```python
from build123d import *

# Parameters (mm, degrees)
BOSS_EXTRUDE1_DEPTH            = 50
SKETCH2_R                      = 7.6
SKETCH2_R_2                    = 4.75
SKETCH2_R_3                    = 1.55
SKETCH2_R_4                    = 1.05
CUT_EXTRUDE1_DEPTH             = 116.876011322
CUT_EXTRUDE2_DEPTH             = 5.5
SKETCH4_R                      = 11
CUT_EXTRUDE3_DEPTH             = 29
CUT_EXTRUDE4_DEPTH             = 5
CUT_EXTRUDE5_DEPTH             = 2.5
SKETCH7_R                      = 4.1
SKETCH7_R_2                    = 1.6
SKETCH7_W                      = 12
SKETCH7_H                      = 24
CUT_EXTRUDE6_DEPTH             = 116.876011322
CUT_EXTRUDE7_DEPTH             = 35
SKETCH9_W                      = 17
SKETCH9_H                      = 16
CUT_EXTRUDE8_DEPTH             = 48
CUT_EXTRUDE9_REACH             = 117.876
SKETCH10_W                     = 37
SKETCH10_H                     = 8
CUT_EXTRUDE9_DIRECTION_2_DEPTH = 116.876011322
CUT_EXTRUDE10_REACH            = 115.716
SKETCH11_W                     = 18.5
SKETCH11_H                     = 8
FILLET1_R                      = 8


with BuildPart() as part:
    # Sketch1 → Boss-Extrude1 (new body)
    with BuildSketch(Plane(origin=(0, 0, 0), x_dir=(0, 0, -1), z_dir=(1, 0, 0))):
        Polygon((0, 0), (0, 30), (5, 30), (5, 35), (-98.5, 35), (-98.5, 0), align=None)
    extrude(amount=BOSS_EXTRUDE1_DEPTH)

    # Sketch2 → Cut-Extrude1 (cut, through all)
    with BuildSketch(Plane(origin=(0, 35, 0), x_dir=(1, 0, 0), z_dir=(0, 1, 0))):
        with Locations(Location((36.5, -48.5, 0), (0, 0, 270))):
            Circle(SKETCH2_R)
        with Locations(Location((13.5, -48.5, 0), (0, 0, 270))):
            Circle(SKETCH2_R_2)
        with Locations(Location((36.5, -36.25, 0), (0, 0, 270))):
            Circle(SKETCH2_R_3)
        with Locations(Location((36.5, -60.75, 0), (0, 0, 270))):
            Circle(SKETCH2_R_3)
        with Locations(Location((19.156854249, -42.843145751, 0), (0, 0, 270))):
            Circle(SKETCH2_R_4)
        with Locations(Location((19.156854249, -54.156854249, 0), (0, 0, 270))):
            Circle(SKETCH2_R_4)
        with Locations(Location((7.843145751, -54.156854249, 0), (0, 0, 270))):
            Circle(SKETCH2_R_4)
        with Locations(Location((7.843145751, -42.843145751, 0), (0, 0, 270))):
            Circle(SKETCH2_R_4)
    extrude(amount=-CUT_EXTRUDE1_DEPTH, mode=Mode.SUBTRACT)

    # Sketch3 → Cut-Extrude2 (cut)
    with BuildSketch(Plane(origin=(0, 35, 0), x_dir=(1, 0, 0), z_dir=(0, 1, 0))):
        with BuildLine():
            Line((25.9, -36.381831822), (25.9, -60.618168178))
            ThreePointArc((25.9, -60.618168178), (36.5, -64.6), (47.1, -60.618168178))
            Line((47.1, -60.618168178), (47.1, -36.381831822))
            ThreePointArc((47.1, -36.381831822), (36.5, -32.4), (25.9, -36.381831822))
        make_face()
    extrude(amount=-CUT_EXTRUDE2_DEPTH, mode=Mode.SUBTRACT)

    # Sketch4 → Cut-Extrude3 (cut)
    with BuildSketch(Plane.XZ):
        with Locations(Location((13.5, 48.5, 0), (0, 0, 270))):
            Circle(SKETCH4_R)
    extrude(amount=-CUT_EXTRUDE3_DEPTH, mode=Mode.SUBTRACT)

    # Sketch5 → Cut-Extrude4 (cut)
    with BuildSketch(Plane.XZ):
        Polygon((39.725, 60.75), (38.1125, 63.542931927), (34.8875, 63.542931927), (33.275, 60.75), (34.8875, 57.957068073), (38.1125, 57.957068073), align=None)
        Polygon((38.1125, 39.042931927), (34.8875, 39.042931927), (33.275, 36.25), (34.8875, 33.457068073), (38.1125, 33.457068073), (39.725, 36.25), align=None)
    extrude(amount=-CUT_EXTRUDE4_DEPTH, mode=Mode.SUBTRACT)

    # Sketch6 → Cut-Extrude5 (cut)
    with BuildSketch(Plane(origin=(0, 35, 0), x_dir=(1, 0, 0), z_dir=(0, 1, 0))):
        Polygon((21.388142908, -42.245273756), (19.754726244, -40.611857092), (17.523437585, -41.209729086), (16.925565591, -43.441017745), (18.558982255, -45.074434409), (20.790270914, -44.476562415), align=None)
        Polygon((21.388142908, -54.754726244), (20.790270914, -52.523437585), (18.558982255, -51.925565591), (16.925565591, -53.558982255), (17.523437585, -55.790270914), (19.754726244, -56.388142908), align=None)
        Polygon((7.245273756, -56.388142908), (9.476562415, -55.790270914), (10.074434409, -53.558982255), (8.441017745, -51.925565591), (6.209729086, -52.523437585), (5.611857092, -54.754726244), align=None)
        Polygon((5.611857092, -42.245273756), (6.209729086, -44.476562415), (8.441017745, -45.074434409), (10.074434409, -43.441017745), (9.476562415, -41.209729086), (7.245273756, -40.611857092), align=None)
    extrude(amount=-CUT_EXTRUDE5_DEPTH, mode=Mode.SUBTRACT)

    # Sketch7 → Cut-Extrude6 (cut, through all)
    with BuildSketch(Plane(origin=(50, 0, 0), x_dir=(0, 0, -1), z_dir=(1, 0, 0))):
        with Locations((-8.5, 26)):
            Circle(SKETCH7_R)
        with Locations((-88.5, 26)):
            Circle(SKETCH7_R)
        with Locations((-88.5, 16)):
            Circle(SKETCH7_R_2)
        with Locations((-8.5, 16)):
            Circle(SKETCH7_R_2)
        with Locations((-68.5, 30)):
            Circle(SKETCH7_R_2)
        with Locations((-68.5, 5)):
            Circle(SKETCH7_R_2)
        with Locations((-24, 15)):
            Rectangle(SKETCH7_W, SKETCH7_H)
    extrude(amount=-CUT_EXTRUDE6_DEPTH, mode=Mode.SUBTRACT)

    # Sketch8 → Cut-Extrude7 (cut)
    with BuildSketch(Plane.ZY):
        Polygon((11.725, 16), (10.1125, 18.792931927), (6.8875, 18.792931927), (5.275, 16), (6.8875, 13.207068073), (10.1125, 13.207068073), align=None)
        Polygon((65.275, 30), (66.8875, 27.207068073), (70.1125, 27.207068073), (71.725, 30), (70.1125, 32.792931927), (66.8875, 32.792931927), align=None)
        Polygon((65.275, 5), (66.8875, 2.207068073), (70.1125, 2.207068073), (71.725, 5), (70.1125, 7.792931927), (66.8875, 7.792931927), align=None)
        Polygon((85.275, 16), (86.8875, 13.207068073), (90.1125, 13.207068073), (91.725, 16), (90.1125, 18.792931927), (86.8875, 18.792931927), align=None)
    extrude(amount=-CUT_EXTRUDE7_DEPTH, mode=Mode.SUBTRACT)

    # Sketch9 → Cut-Extrude8 (cut)
    with BuildSketch(Plane(origin=(50, 0, 0), x_dir=(0, 0, -1), z_dir=(1, 0, 0))):
        with Locations((-24, 13)):
            Rectangle(SKETCH9_W, SKETCH9_H)
    extrude(amount=-CUT_EXTRUDE8_DEPTH, mode=Mode.SUBTRACT)

    # Sketch10 → Cut-Extrude9 (cut, up to next)
    with BuildSketch(Plane.XZ, mode=Mode.PRIVATE) as cut_extrude9_sk1:
        with Locations((25, 24)):
            Rectangle(SKETCH10_W, SKETCH10_H)
    cut_extrude9_tool1 = extrude(cut_extrude9_sk1.sketch, amount=-CUT_EXTRUDE9_REACH, mode=Mode.PRIVATE) & part.part
    add(cut_extrude9_tool1.solids().sort_by_distance((25, 0, 24))[0], mode=Mode.SUBTRACT)

    # Sketch10 → Cut-Extrude9 direction 2 (cut)
    with BuildSketch(Plane.XZ):
        with Locations((25, 24)):
            Rectangle(SKETCH10_W, SKETCH10_H)
    extrude(amount=CUT_EXTRUDE9_DIRECTION_2_DEPTH, mode=Mode.SUBTRACT)

    # Sketch11 → Cut-Extrude10 (cut, up to next)
    with BuildSketch(Plane.XZ.offset(-27), mode=Mode.PRIVATE) as cut_extrude10_sk1:
        with Locations((15.75, 24)):
            Rectangle(SKETCH11_W, SKETCH11_H)
    cut_extrude10_tool1 = extrude(cut_extrude10_sk1.sketch, amount=-CUT_EXTRUDE10_REACH, mode=Mode.PRIVATE) & part.part
    add(cut_extrude10_tool1.solids().sort_by_distance((15.75, 27, 24))[0], mode=Mode.SUBTRACT)

    # Fillet1
    fillet1_edges = [part.edges().sort_by_distance(p)[0] for p in [
        (25, 35, 98.5),
    ]]
    fillet(fillet1_edges, radius=FILLET1_R)


solid = part.part
```
Design review of the part built by this model. Coordinates are the model's own, in mm. A direction names the side the tool comes from. Round coordinates to 2 decimals unless told otherwise and drop trailing zeros. Order: outer loops, then holes, each group sorted by start corner. A loop starts at its lowest first (then second) coordinate and runs counter-clockwise, first axis right, second up. Notation, with made-up numbers: (46, 22) - (53, 22) arc R25 ccw to (53, 50) - close; hole circle Ø10 at (75.25, 29). An arc over 180 degrees is marked (long way). One line per question, with ' | ' between items.
Item 1: Machinability: for faces 1 (the face through (38.907, 2.465, 34.834)), 2 (the face through (25, 31, 24)), 3 (the face through (26, 13, 15.5)), 4 (the face through (18.655, 33.768, 40.907)), 5 (the face through (35, 31, 70)), which of the approach directions +Z, -Z, +X, -X, +Y, -Y give a long, thin tool a straight path to every point of the face, cutting with its end or side? Answer none if there is none.
Checks:
face 1: -Y | face 2: +Y, -Y | face 3: +X | face 4: +Y | face 5: -X
Item 2: Wall thickness on line 1 (Y direction, x = 26.5, z = 68.5); line 2 (Z direction, x = 28.5, y = 12); line 3 (Z direction, x = 10, y = 14): over which ranges is each line inside the solid? List them lowest first. Write a range as [from, to].
Checks:
line 1: [0, 2.21], [7.79, 27.21], [32.79, 35] | line 2: [0, 15.5], [32.5, 98.5] | line 3: [0, 6.43], [10.57, 15.5], [32.5, 38.07], [58.93, 86.43], [90.57, 98.5]
Item 3: Take a section at A-A, the plane z = 68.5. Write out the cut boundary in (x, y), then the cut area to 3 significant figures.
Checks:
outline: (0, 0) - (50, 0) - (50, 3.4) - (35, 3.4) - (35, 2.21) - (0, 2.21) - close; (0, 7.79) - (35, 7.79) - (35, 6.6) - (50, 6.6) - (50, 28.4) - (35, 28.4) - (35, 27.21) - (0, 27.21) - close; (0, 32.79) - (35, 32.79) - (35, 31.6) - (50, 31.6) - (50, 35) - (0, 35) - close | area: 1,260 mm²
Item 4: Take a section at C-C, the plane x = 36.5. Give the number of separate pieces and of enclosed holes in the cut face, then the cut area to 3 significant figures.
Checks:
separate pieces: 4 | enclosed holes: 6 | area: 2,100 mm²
Item 5: Draft analysis for pull direction Z (two halves, no side actions). For faces 6 (the face through (25, 14, 98.5)), 7 (the face through (25, 15, 0)), 8 (the face through (17.26, 17.38, 90.93)), state which applies: +Z half, -Z half, draft (parallel to the pull), parting line (faces both ways), or undercut.
Checks:
face 6: +Z half | face 7: -Z half | face 8: undercut
Item 6: For P1, Ø4, axis at x = 40.5, y = 22, coming from the -Z side; P2, Ø4, axis at y = 21.5, z = 45, coming from the -X side; P3, Ø2.5, axis at y = 30, z = 68.5, coming from the -X side; P4, Ø3.5, axis at x = 7.84, z = 42.84, coming from the -Y side, all flat-tipped, find the tip position at first contact; note any pin that passes through.
Checks:
P1: z = 0 | P2: x = 0 | P3: through | P4: y = 29
Item 7: Take a section at D-D, the plane z = 88.5. Write out the cut boundary in (x, y).
Checks:
outline: (0, 0) - (50, 0) - (50, 14.4) - (35, 14.4) - (35, 13.21) - (0, 13.21) - close; (0, 18.79) - (35, 18.79) - (35, 17.6) - (50, 17.6) - (50, 21.9) - (0, 21.9) - close; (0, 30.1) - (50, 30.1) - (50, 35) - (0, 35) - close
Item 8: Take a section at B-B, the plane y = 9.5. Write out the cut boundary in (x, z), then the cut area to 3 significant figures.
Checks:
outline: (0, 0) - (50, 0) - (50, 15.5) - (2, 15.5) - (2, 18) - (0, 18) - close; (0, 30) - (2, 30) - (2, 32.5) - (50, 32.5) - (50, 98.5) - (0, 98.5) - close; hole circle Ø22 at (13.5, 48.5); hole circle Ø15.2 at (36.5, 48.5); hole circle Ø3.1 at (36.5, 36.25); hole circle Ø3.1 at (36.5, 60.75) | area: 3,510 mm²
